Input: part model. Units: mm. Frame: model coordinates. Give positions to 0.01 mm unless a question says otherwise; leave off trailing zeros. Loops run counter-clockwise (first coordinate to the right, second up) from the corner with the lowest first, then second, coordinate; pieces in that order, holes last. Notation, with made-up numbers: M -21.5,23 L 25.5,23 A12 cw 25.5,43 Z; hole C 21,4.5 d9. An arc over 180 degrees is marked long. Answer as a JSON object with one key per item and string values. Group by question number.
1) Section query C-C on x = -120. Return loops of the section in (y, z), plus the area to 3 significant figures.
2) Ray query, L1, parallel to Y at x = -120, z = 3.5; L2, parallel to X at y = 72.5, z = 4; L3, parallel to X at y = -68, z = 1.5. Return the intervals inside material, ascending.
3) Section query B-B on z = 5. Return loops of the section in (x, y).
4) Section query A-A on y = -75. Return loops of the section in (x, z), plus the area to 3 significant figures.
5) First-contact query: P1, Ø20.5, axis at x = -120, y = 72.5, coming from the -Z side. Flat tip, straight axial feed; report the tip coordinate or a pass-through.
6) Draft query along Y for faces 1 (the cylindrical face through (122.493, -63.773, 6.077)), 2 (the flat face through (-2, 125, 6)), 3 (the flat face through (170, -2, 6)), 4 (the cylindrical face through (-117.507, 83.727, 6.077)). Return one class per face: +Y half, -Y half, draft (parallel to the pull), parting line (faces both ways), or undercut.
from build123d import *

# Parameters (mm, degrees)
F0_W     = 340
F0_H     = 250
F1_DEPTH = 12
F2_D     = 23
F3_SIZE  = 0.5


with BuildPart() as f1:
    # F0 (on Top) → F1 (new body)
    with BuildSketch(Plane.XY):
        Rectangle(F0_W, F0_H)
    extrude(amount=F1_DEPTH)

    # F2 (through all)
    with Locations(Plane(origin=(0, 0, 0), x_dir=(1, 0, 0), z_dir=(0, 0, -1))):
        with Locations((120, -72.5), (120, 75), (-120, 75), (-120, -72.5)):
            Hole(F2_D / 2)

    # F3
    f3_edges = [f1.edges().sort_by_distance(p)[0] for p in [
        (170, 0, 12),
        (0, -125, 12),
        (0, 125, 12),
        (-170, 0, 12),
        (-131.5, -75, 12),
        (108.5, -75, 12),
        (-131.5, 72.5, 12),
        (108.5, 72.5, 12),
        (170, 0, 0),
        (0, -125, 0),
        (0, 125, 0),
        (-170, 0, 0),
        (-131.5, -75, 0),
        (108.5, -75, 0),
        (-131.5, 72.5, 0),
        (108.5, 72.5, 0),
    ]]
    chamfer(f3_edges, length=F3_SIZE)


solid = f1.part
Output:
{
 "1": {"outline": "M -125,0.5 L -124.5,0 L -87,0 L -86.5,0.5 L -86.5,11.5 L -87,12 L -124.5,12 L -125,11.5 Z; M -63.5,0.5 L -63,0 L 60.5,0 L 61,0.5 L 61,11.5 L 60.5,12 L -63,12 L -63.5,11.5 Z; M 84,0.5 L 84.5,0 L 124.5,0 L 125,0.5 L 125,11.5 L 124.5,12 L 84.5,12 L 84,11.5 Z", "area": "2,450 mm^2"},
 "2": {"L1": "y = -125 to -86.5, -63.5 to 61, 84 to 125", "L2": "x = -170 to -131.5, -108.5 to 108.5, 131.5 to 170", "L3": "x = -170 to -129.12, -110.88 to 110.88, 129.12 to 170"},
 "3": {"outline": "M -170,-125 L 170,-125 L 170,125 L -170,125 Z; hole C -120,-75 d23; hole C -120,72.5 d23; hole C 120,-75 d23; hole C 120,72.5 d23"},
 "4": {"outline": "M -170,0.5 L -169.5,0 L -132,0 L -131.5,0.5 L -131.5,11.5 L -132,12 L -169.5,12 L -170,11.5 Z; M -108.5,0.5 L -108,0 L 108,0 L 108.5,0.5 L 108.5,11.5 L 108,12 L -108,12 L -108.5,11.5 Z; M 131.5,0.5 L 132,0 L 169.5,0 L 170,0.5 L 170,11.5 L 169.5,12 L 132,12 L 131.5,11.5 Z", "area": "3,530 mm^2"},
 "5": {"P1": "passes through"},
 "6": {"face 1": "undercut", "face 2": "+Y half", "face 3": "draft", "face 4": "undercut"}
}
